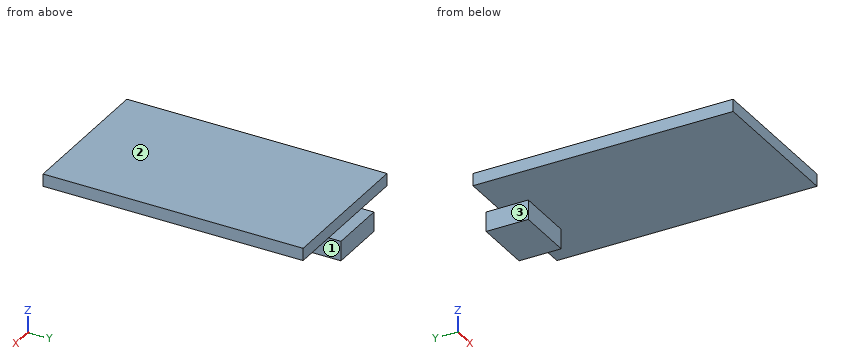
from build123d import *

# Parameters (mm, degrees)
SKETCH1_W           = 20.4
SKETCH1_H           = 35.8
BOSS_EXTRUDE1_DEPTH = 1.7
SKETCH2_W           = 8
SKETCH2_H           = 5.8
BOSS_EXTRUDE2_DEPTH = 2.7


with BuildPart() as part:
    # Sketch1 → Boss-Extrude1 (new body)
    with BuildSketch(Plane.XY):
        with Locations((0, -17.9)):
            Rectangle(SKETCH1_W, SKETCH1_H)
    extrude(amount=-BOSS_EXTRUDE1_DEPTH)

    # Sketch2 → Boss-Extrude2 (add)
    with BuildSketch(Plane(origin=(0, 0, -1.7), x_dir=(-1, 0, 0), z_dir=(0, 0, -1))):
        with Locations((0, -1.2)):
            Rectangle(SKETCH2_W, SKETCH2_H)
    extrude(amount=BOSS_EXTRUDE2_DEPTH)


solid = part.part
For this review, take the finished solid that the model builds, in its own axes (mm). Face numbers are marked on the shaded views. A direction names the side the tool comes from. Give positions to 0.01 mm unless a question says otherwise; leave off trailing zeros. Loops run counter-clockwise (first coordinate to the right, second up) from the corner with the lowest first, then second, coordinate; pieces in that order, holes last.
Item 1: Tool access review of the marked faces 1, 2 and 3: name each direction out of +Z, -Z, +X, -X, +Y, -Y from which nothing blocks a thin tool from reaching the whole face with its end or side.
Item 2: Insertion check: pin 1 (10 mm diameter, centred on x = -1.5, y = -21, fed in from -Z); pin 2 (1.4 mm diameter, centred on x = 4.5, z = -0.5, fed in from +Y); pin 3 (2 mm diameter, centred on y = -1.5, z = -3.5, fed in from +X). Each pin has a flat end and moves straight along its axis. Give the tip position at first contact, or say it passes through.
Item 3: Take a section at D-D, the plane z = -2.5. State the section outline as (x, y) points, and give its area (3 significant figures).
Item 4: For line 1 along Y through (x, z) = (-1.5, -0.85); line 2 along Z through (x, y) = (0.25, -15); line 3 along Y through (x, z) = (2.5, -3.5), list the stretches that pass through material, from the lowest coordinate up.
Item 5: Take a section at A-A, the plane x = -2. State the section outline as (y, z) points.
Item 6: Take a section at C-C, the plane z = -0.55. State the section outline as (x, y) points, and give its area (3 significant figures).
Item 7: Take a section at B-B, the plane y = -1. State the section outline as (x, z) points, and give its area (3 significant figures).
Calculated:
1. face 1: -Z, +X, +Y, -Y
1. face 2: +Z, +X, -X, +Y, -Y
1. face 3: -Z, -X, +Y, -Y
2. pin 1: stops at z = -1.7
2. pin 2: stops at y = 0
2. pin 3: stops at x = 4
3. outline: (-4, -4.1) - (4, -4.1) - (4, 1.7) - (-4, 1.7) - close
3. area: 46.4 mm2
4. line 1: y = -35.8 to 0
4. line 2: z = -1.7 to 0
4. line 3: y = -4.1 to 1.7
5. outline: (-35.8, -1.7) - (-4.1, -1.7) - (-4.1, -4.4) - (1.7, -4.4) - (1.7, -1.7) - (0, -1.7) - (0, 0) - (-35.8, 0) - close
6. outline: (-10.2, -35.8) - (10.2, -35.8) - (10.2, 0) - (-10.2, 0) - close
6. area: 730 mm2
7. outline: (-10.2, -1.7) - (-4, -1.7) - (-4, -4.4) - (4, -4.4) - (4, -1.7) - (10.2, -1.7) - (10.2, 0) - (-10.2, 0) - close
7. area: 56.3 mm2
